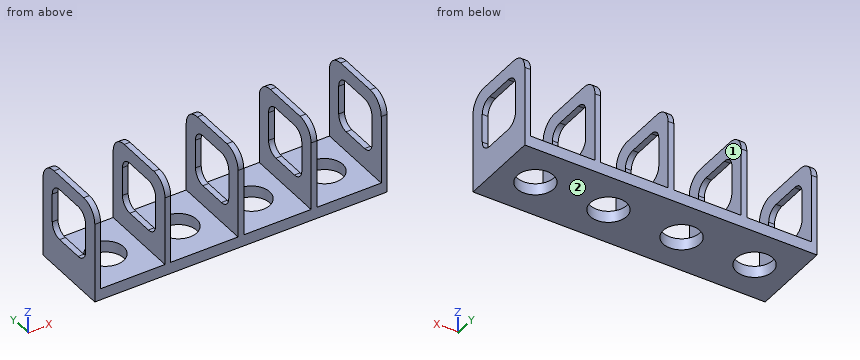
Autodesk Inventor part; units mm, degrees
ref_plane "YZ Plane" through (0, 0, 0) normal (1, 0, 0) x (0, 1, 0)
ref_plane "XZ Plane" through (0, 0, 0) normal (0, 1, 0) x (-1, 0, 0)
ref_plane "XY Plane" through (0, 0, 0) normal (0, 0, 1) x (1, 0, 0)
sketch "Sketch1" plane through (0, 0, 0) normal (0, 0, 1) x (1, 0, 0)
  circle A0 centre (-19.0795, 0) radius 3.175
  circle A1 centre (-6.3598, 0) radius 3.175
  circle A2 centre (6.3597, 0) radius 3.175
  circle A3 centre (19.0795, 0) radius 3.175
  line L0 (25, -19) -> (25, 19)
  line L1 (-25, 19) -> (-25, -19)
  line L2 (-19.0795, 0) -> (-6.3598, 0)
  line L3 (-6.3598, 0) -> (-12.7197, 0)
  line L4 (-19.0795, 0) -> (-25.4395, 0)
  line L5 (19.0795, 0) -> (25.4395, 0)
  line L6 (-12.2197, 7) -> (-12.2197, -7)
  line L7 (-12.2197, -7) -> (-13.2197, -7)
  line L8 (-13.2197, -7) -> (-13.2197, 7)
  line L9 (-13.2197, 7) -> (-12.2197, 7)
  line L10 (-12.2197, 7) -> (-13.2197, -7) construction
  line L11 (-12.2197, -7) -> (-13.2197, 7) construction
  line L12 (-25.4395, 0) -> (-25.9395, 0)
  line L13 (-25.9395, 0) -> (-25.9395, 7)
  line L14 (25.4395, 0) -> (25.9395, 0)
  line L15 (25.9395, 0) -> (25.9395, -7)
  line L16 (-25.9395, 7) -> (25.9395, 7)
  line L17 (25.9395, 7) -> (25.9395, -7)
  line L18 (25.9395, -7) -> (-25.9395, -7)
  line L19 (-25.9395, -7) -> (-25.9395, 7)
  point P0 (0, 0)
  point P1 (-25, 7)
  point P2 (-25, -7)
  point P3 (25, -7)
  point P4 (25, 7)
  dimension "d0" = 6.36
  dimension "d1" = 6.36
  dimension "d2" = 14
  dimension "d3" = 1
  dimension "d4" = 0.5
  dimension "d5" = 7
  dimension "d6" = 0.5
  dimension "d7" = 7
extrude "Extrusion1" add sketch "Sketch1" along normal blind 2 contours L2 L8 L18 L1 L4 A0 | A0 L4 L1 L16 L8 L2 | L8 L9 L6 L2 | L2 L6 L7 L8 | L6 L16 L0 L18
sketch "Sketch2" plane through (0, 0, 2) normal (0, 0, 1) x (1, 0, 0)
  line L0 (-25, 7) -> (-24, 7)
  line L1 (25, 7) -> (-25, 7)
  circle A0 centre (-19.0795, 0) radius 3.175
  circle A1 centre (-6.3598, 0) radius 3.175
  line L2 (-19.0795, 0) -> (-6.3598, 0)
  line L3 (-13.2197, 7) -> (-13.2197, -7)
  line L4 (-13.2197, -7) -> (-12.2197, -7)
  line L5 (-12.2197, -7) -> (-12.2197, 7)
  line L6 (-12.2197, 7) -> (-13.2197, 7)
  line L7 (-13.2197, 7) -> (-12.2197, -7) construction
  line L8 (-13.2197, -7) -> (-12.2197, 7) construction
  line L9 (-0.5, 7) -> (-0.5, -7)
  line L10 (-0.5, -7) -> (0.5, -7)
  line L11 (0.5, -7) -> (0.5, 7)
  line L12 (0.5, 7) -> (-0.5, 7)
  line L13 (-0.5, 7) -> (0.5, -7) construction
  line L14 (-0.5, -7) -> (0.5, 7) construction
  circle A2 centre (6.3597, 0) radius 3.175
  circle A3 centre (19.0795, 0) radius 3.175
  line L15 (6.3597, 0) -> (19.0795, 0)
  line L16 (12.2196, 7) -> (12.2196, -7)
  line L17 (12.2196, -7) -> (13.2196, -7)
  line L18 (13.2196, -7) -> (13.2196, 7)
  line L19 (13.2196, 7) -> (12.2196, 7)
  line L20 (12.2196, 7) -> (13.2196, -7) construction
  line L21 (12.2196, -7) -> (13.2196, 7) construction
  line L22 (-24, 7) -> (-25, 7)
  line L23 (-25, 7) -> (-25, -7)
  line L24 (-25, -7) -> (-24, -7)
  line L25 (25, -7) -> (25, 7)
  line L26 (-25, -7) -> (25, -7)
  line L27 (25, 7) -> (24, 7)
  line L28 (24, 7) -> (24, -7)
  line L29 (24, -7) -> (25, -7)
  line L30 (25, -7) -> (25, 7)
  line L31 (-12.7197, 0) -> (-24.4397, 0)
  line L32 (-24.4397, 0) -> (-24.4397, 7)
  line L33 (-24.4397, 7) -> (-25.4397, 7)
  line L34 (-25.4397, 7) -> (-25.4397, -7)
  line L35 (-25.4397, -7) -> (-24.4397, -7)
  line L36 (-24.4397, -7) -> (-24.4397, 7)
  line L37 (0, 7) -> (0, -7)
  line L38 (25.4397, 7) -> (25.4397, -7)
  line L39 (25.4397, 7) -> (24.4397, 7)
  line L40 (24.4397, 7) -> (24.4397, -7)
  line L41 (24.4397, -7) -> (25.4397, -7)
  line L42 (25.4397, -7) -> (25.4397, 7)
  point P0 (0, 0)
  point P1 (12.7196, 0)
  dimension "d10" = 1
  dimension "d11" = 1
  dimension "d12" = 1
  dimension "d13" = 1
  dimension "d14" = 1
  dimension "d27" = 11.72
  dimension "d28" = 1
  dimension "d29" = 1
extrude "Extrusion2" add sketch "Sketch2" along normal blind 15 contours L0 L32 L36 L24 L23 | L23 L35 L34 L33 | L1 L5 L2 L3 | L2 L5 L4 L3 | L1 L37 L10 L9 | L1 L11 L10 L37 | L1 L18 L15 L16 | L15 L18 L17 L16 | L1 L25 L26 L40 | L39 L38 L41 L25
sketch "Sketch3" plane through (-25, -7, 0) normal (-1, 0, 0) x (0, 0, 1)
  line L0 (2, 14) -> (2, 0)
  line L1 (0, 14) -> (2, 14)
  line L2 (0, 0) -> (2, 0)
  line L3 (14, 14) -> (3, 14)
  line L4 (3, 14) -> (3, 0)
  line L5 (3, 0) -> (14, 0)
  line L6 (17, 3) -> (17, 11)
  line L7 (7.5, 11.5) -> (12.5, 11.5)
  line L8 (14.5, 9.5) -> (14.5, 4.5)
  line L9 (12.5, 2.5) -> (7.5, 2.5)
  line L10 (5.5, 4.5) -> (5.5, 9.5)
  line L11 (5.5, 11.5) -> (14.5, 2.5) construction
  line L12 (14.5, 11.5) -> (5.5, 2.5) construction
  arc A0 (17, 11) -> (14, 14) centre (14, 11) ccw
  arc A1 (14, 0) -> (17, 3) centre (14, 3) ccw
  arc A2 (14.5, 9.5) -> (12.5, 11.5) centre (12.5, 9.5) ccw
  arc A3 (12.5, 2.5) -> (14.5, 4.5) centre (12.5, 4.5) ccw
  arc A4 (7.5, 11.5) -> (5.5, 9.5) centre (7.5, 9.5) ccw
  arc A5 (5.5, 4.5) -> (7.5, 2.5) centre (7.5, 4.5) ccw
  line L13 (17, 14) -> (17, 0)
  line L14 (0, 14) -> (2, 14)
  point P0 (0, 7)
  point P1 (10, 7)
  dimension "d18" = 14
  dimension "d19" = 9
  dimension "d20" = 9
  dimension "d21" = 3
  dimension "d22" = 3
  dimension "d23" = 2
extrude "Extrusion3" cut sketch "Sketch3" against normal through all contours L7 A2 L8 A3 L9 A5 L10 A4
sketch "Sketch4" plane through (-25.4397, -7, 2) normal (-1, 0, 0) x (0, 0, 1)
  line L0 (0, 14) -> (0, 0)
  line L1 (-2, 14) -> (0, 14)
  line L2 (-2, 0) -> (0, 0)
  line L3 (12, 14) -> (1, 14)
  line L4 (1, 14) -> (1, 0)
  line L5 (1, 0) -> (12, 0)
  line L6 (15, 3) -> (15, 11)
  line L7 (5.5, 11.5) -> (10.5, 11.5)
  line L8 (12.5, 9.5) -> (12.5, 4.5)
  line L9 (10.5, 2.5) -> (5.5, 2.5)
  line L10 (3.5, 4.5) -> (3.5, 9.5)
  line L11 (3.5, 11.5) -> (12.5, 2.5) construction
  line L12 (12.5, 11.5) -> (3.5, 2.5) construction
  arc A0 (15, 11) -> (12, 14) centre (12, 11) ccw
  arc A1 (12, 0) -> (15, 3) centre (12, 3) ccw
  arc A2 (12.5, 9.5) -> (10.5, 11.5) centre (10.5, 9.5) ccw
  arc A3 (10.5, 2.5) -> (12.5, 4.5) centre (10.5, 4.5) ccw
  arc A4 (5.5, 11.5) -> (3.5, 9.5) centre (5.5, 9.5) ccw
  arc A5 (3.5, 4.5) -> (5.5, 2.5) centre (5.5, 4.5) ccw
  line L13 (15, 14) -> (15, 0)
  line L14 (-2, 14) -> (0, 14)
  line L15 (-2, 0) -> (0, 0)
  line L16 (-2, 0) -> (15, 0)
  line L17 (15, 0) -> (15, 14)
  line L18 (15, 14) -> (-2, 14)
  line L19 (-2, 14) -> (-2, 0)
  point P0 (-2, 7)
  point P1 (-2, 7)
  point P2 (15, 0)
  point P3 (8, 7)
  point P4 (12, 0)
  dimension "d30" = 14
  dimension "d31" = 9
  dimension "d32" = 9
  dimension "d33" = 3
  dimension "d34" = 3
  dimension "d35" = 2
extrude "Extrusion4" cut sketch "Sketch4" against normal through all contours L18 L13 A0 | A1 L13 L16 | L7 A2 L8 A3 L9 A5 L10 A4
sketch "Sketch5" plane through (-25, -7, 0) normal (-1, 0, 0) x (0, 0, 1)
  line L0 (2, 14) -> (2, 0)
  line L1 (0, 14) -> (2, 14)
  line L2 (0, 0) -> (0, 14)
  line L3 (2, 14) -> (0, 14)
  line L4 (0, 14) -> (0, 0)
  line L5 (0, 0) -> (2, 0)
  line L6 (2, 0) -> (2, 14)
  point P0 (0, 7)
  point P1 (2, 0)
extrude "Extrusion5" add sketch "Sketch5" along normal up to surface (0.4397 mm away)
sketch "Sketch6" plane through (25, -7, 0) normal (1, 0, 0) x (0, 0, -1)
  line L0 (-2, 0) -> (-2, 14)
  line L1 (0, 0) -> (0, 14)
  line L2 (0, 0) -> (0, 14)
  line L3 (0, 14) -> (-2, 14)
  line L4 (-2, 0) -> (-2, 14)
  line L5 (0, 0) -> (-2, 0)
  point P0 (0, 7)
extrude "Extrusion6" add sketch "Sketch6" along normal up to surface (0.4397 mm away)
properties part number "protector_small1x1"
CAD build for the part. Positions are in the model's coordinates, mm. Face numbers are marked on the shaded views. A direction names the side the tool comes from. Coordinates: 2 decimals unless noted, no trailing zeros. Loops run counter-clockwise (first coordinate to the right, second up) from the corner with the lowest first, then second, coordinate; pieces in that order, holes last. Notation, with made-up numbers: (21.25, -23.5) - (52.25, -23.5) arc R21 cw to (52.25, -0.5) - close; hole circle Ø3 at (87.5, -31.5). An arc over 180 degrees is marked (long way). Use CSV: the item, a comma, the result in double quotes. Start each with the question number.
Q1. Cut at D-D, the plane z = 10.75. State how many separate pieces and enclosed holes the cut face has, then the cut area to 3 significant figures.
Q2. Probe probe 1 along X at (y, z) = (4, 4.25); probe 2 along Z at (x, y) = (21.5, -2.75); probe 3 along Y at (x, z) = (9, 1.75). List the from-to ranges inside material, lowest first. Write a range as from..to.
Q3. Drop a flat-ended pin along its axis: P1, Ø5.5, axis at x = -19.08, y = 0, coming from the +Z side. Give the stop position or say it passes through.
Q4. Cut at A-A, the plane z = 3.75. List the corners of the cut face in (x, y), then the cut area to 3 significant figures.
Q5. 3-axis set-ups, long thin cutter, end or side, ignore diameter. For the marked faces 1 and 2: which of +Z, -Z, +X, -X, +Y, -Y reach the whole face in a straight line?
Q6. Cut at C-C, the plane y = -6. List the corners of the cut face in (x, z), then the cut area to 3 significant figures.
Q7. Cut at B-B, the plane x = 9. List the corners of the cut face in (y, z).
Here are the results:
1,separate pieces,"10"
1,enclosed holes,"0"
1,area,"25.0 mm2"
2,probe 1,"-25.44..-24.44, -13.22..-12.22, -0.5..0.5, 12.22..13.22, 24.44..25.44"
2,probe 2,"0..2"
2,probe 3,"-7..-1.76, 1.76..7"
3,P1,"through"
4,outline,"(-25.44, -7) - (-24.44, -7) - (-24.44, 7) - (-25.44, 7) - close; (-13.22, -7) - (-12.22, -7) - (-12.22, 7) - (-13.22, 7) - close; (-0.5, -7) - (0.5, -7) - (0.5, 7) - (-0.5, 7) - close; (12.22, -7) - (13.22, -7) - (13.22, 7) - (12.22, 7) - close; (24.44, -7) - (25.44, -7) - (25.44, 7) - (24.44, 7) - close"
4,area,"70.0 mm2"
5,face 1,"+Z, +Y, -Y"
5,face 2,"-Z, +X, -X, +Y, -Y"
6,outline,"(-25.44, 0) - (25.44, 0) - (25.44, 16.24) - (24.44, 16.24) - (24.44, 2) - (13.22, 2) - (13.22, 16.24) - (12.22, 16.24) - (12.22, 2) - (0.5, 2) - (0.5, 16.24) - (-0.5, 16.24) - (-0.5, 2) - (-12.22, 2) - (-12.22, 16.24) - (-13.22, 16.24) - (-13.22, 2) - (-24.44, 2) - (-24.44, 16.24) - (-25.44, 16.24) - close"
6,area,"173 mm2"
7,outline,"(-7, 0) - (-1.76, 0) - (-1.76, 2) - (-7, 2) - close; (1.76, 0) - (7, 0) - (7, 2) - (1.76, 2) - close"
